The listing builds one solid part. Answer for the finished solid, in the listing's coordinates (mm). A direction names the side the tool comes from. Give positions to 0.01 mm unless a question says otherwise; leave off trailing zeros. Write each loop counter-clockwise with the first axis right and the second up, starting at its lowest first coordinate (ties: lowest second). Pieces come first, ordered by that corner, then holes. Notation, with made-up numbers: M 18.25,20 L 46.25,20 A32 ccw 46.25,57 Z; hole C -15,79 d4. An arc over 180 degrees is marked long. Answer as a JSON object with one key per item and string values.
Autodesk Inventor part; units mm, degrees
ref_plane "MSC_PF1" through (0, 0, 0) normal (1, 0, 0) x (0, 1, 0)
ref_plane "MSC_PT1" through (0, 0, 0) normal (0, 0, -1) x (-1, 0, 0)
ref_plane "YZ Plane" through (0, 0, 0) normal (1, 0, 0) x (0, 1, 0)
sketch "Esquisse1" plane through (0, 0, 0) normal (0, 1, 0) x (-1, 0, 0)
  point P0 (0, 0)
sketch "Esquisse2" plane through (0, 0, 0) normal (0, 0, 1) x (1, 0, 0)
  point P0 (0, 0)
sketch "Esquisse3" plane through (0, 0, 0) normal (0, 0, 1) x (1, 0, 0)
  point P0 (0, 0)
sketch "Esquisse4" plane through (0, 0, 0) normal (0, 1, 0) x (-1, 0, 0)
  line L0 (-3.65, 0) -> (0, 0)
  line L1 (-3.65, -0.45) -> (-3.65, 0)
  line L2 (-1.75, -2.35) -> (-3.65, -0.45)
  line L3 (-1.75, -2.65) -> (-1.75, -2.35)
  line L4 (-1.45, -2.95) -> (-1.75, -2.65)
  line L5 (-1.75, -3.25) -> (-1.45, -2.95)
  line L6 (-1.75, -10) -> (-1.75, -3.25)
  line L7 (0, 0) -> (0, -10)
  line L8 (0, 3.3392) -> (0, -10.7) construction
  line L9 (0, 3.3392) -> (0, -10.7)
  line L10 (0, -13.5078) -> (0, 6.1471)
  line L11 (-1.75, -10) -> (0, -10)
  line L12 (0.73, 0) -> (-4.38, 0)
  dimension "d3" = 3.65
  dimension "d5" = 0.3
  dimension "d7" = 0.3
  dimension "d9" = 0.3
  dimension "d11" = 2.35
  dimension "d13" = 135
  dimension "d17" = 1.45
  dimension "d19" = 0
  dimension "d51" = 1.75
  dimension "d52" = 10
revolve "Révolution1" add sketch "Esquisse4" angle 360 about axis through (0, 0, 3.3392) along (0, 0, -1)
sketch "Esquisse5" plane through (0, 0, 0) normal (0, 1, 0) x (-1, 0, 0)
  line L0 (-2.2, 0) -> (0, 0)
  line L1 (-0.3667, -2.1364) -> (-2.2, 0)
  line L2 (0, -2.1364) -> (-0.3667, -2.1364)
  line L3 (0, 0) -> (0, -2.1364)
  line L4 (-1.75, -2.35) -> (1.75, -2.35) construction
  line L5 (-3.65, 0) -> (3.65, 0)
  line L6 (0, -2.82) -> (0, 0.47)
  dimension "d22" = 2.2
  dimension "d24" = 0.3667
  dimension "d26" = 2.1364
extrude "Extrusion1" cut sketch "Esquisse5" along normal mid plane 0.7333
pattern_circular "RéseauPolaire1" count 4 over 360 about axis through (0, 0, 0) along (0, 0, 1) of "Extrusion1"
sketch "Esquisse7" plane through (0, 0, 0) normal (0, 1, 0) x (-1, 0, 0)
  line L0 (0, -1.175) -> (-2.75, 0)
  line L1 (0, 0) -> (0, -1.175)
  line L2 (-2.75, 0) -> (0, 0)
  line L3 (-1.75, -2.35) -> (1.75, -2.35) construction
  line L4 (0, -2.82) -> (0, 0.47)
  line L5 (-3.65, 0) -> (3.65, 0)
  dimension "d33" = 2.75
  dimension "d35" = 1.175
extrude "Extrusion2" cut sketch "Esquisse7" along normal mid plane 0.7333
pattern_circular "RéseauPolaire2" count 4 over 360 about axis through (0, 0, 0) along (0, 0, 1) of "Extrusion2"
fillet "Congé1" radius 0.6 1 edges at (-1.75, 0, -2.35)
thread "Filetage1"
ref_plane "MSC_PF1" through (0, 0, 0) normal (1, 0, 0) x (0, 1, 0)
ref_plane "MSC_PT1" through (0, 0, 0) normal (0, 0, -1) x (-1, 0, 0)
equation "\"d3\" = 0.5 * Dh"
equation "\"d5\" = msp_x"
equation "\"d7\" = ParA"
equation "\"d9\" = msp_x"
equation "\"d11\" = ParK"
equation "\"d17\" = 0.5 * msp_mdtds"
equation "\"d51\" = 0.5 * NND"
equation "\"d52\" = NLG"
equation "\"d22\" = 0.5 * M"
equation "\"d24\" = 0.0833333 * M"
equation "\"d26\" = 0.909091 * ParK"
equation "\"d27\" = 0.166667 * M"
equation "\"d33\" = 0.625 * M"
equation "\"d35\" = 0.5 * ParK"
equation "\"d36\" = 0.166667 * M"
equation "\"d41\" = 2 * msp_x"
equation "\"PTC\" = 0.6"
equation "\"NLG\" = 10"
equation "\"ParK\" = 2.35"
equation "\"NND\" = 3.5"
equation "\"M\" = 4.4"
equation "\"msp_mdtds\" = NND - PTC"
equation "\"Dh\" = 7.3"
equation "\"msp_x\" = 0.5 * PTC"
equation "\"ParA\" = 0.5 * PTC"
equation "\"r\" = 0.9"
equation "\"THREADDIA\" = NND"
equation "\"TEMPLATE\" = 1.2345"
properties part number "NF EN ISO 7046-2 H - M3.5x10 - 8.8 - H1" material "Acier inoxydable 440C"
1. A cutting plane is placed at A-A, the plane z = -6.75. Give the vertices of the cut face in (x, y).
Verdict:
{"outline": "C 0,0 d3.5"}
2. For faces 4 (the flat face through (0, 0, -10)), 5 (the flat face through (0.01, 1.11, -1.27)), 6 (the cylindrical face through (1.617, -0.67, -6.578)), determine the directions among +Z, -Z, +X, -X, +Y, -Y from which every point of the face is accessible in a straight line to the end or side of a thin tool.
Verdict:
{"face 4": "-Z, +X, -X, +Y, -Y", "face 5": "+Z", "face 6": "-Z"}
3. The mould has two halves that part along X. Classify faces 1 (the flat face through (-0.367, -1, -1)), 2 (the conical face through (-0.441, -1.985, -2.066)), 3 (the flat face through (1, 1, 0)): released by +X, released by -X, zero draft, split by the parting line, or undercut.
Verdict:
{"face 1": "undercut", "face 2": "split by the parting line", "face 3": "zero draft"}
4. Flat-ended cylindrical pins translate along their axes: pin 1 (2.5 mm diameter, centred on x = 2, z = -1.5, fed in from +Y); pin 2 (1.1 mm diameter, centred on y = 2, z = -1, fed in from -X); pin 3 (0.6 mm diameter, centred on x = 0, y = 0, fed in from +Z). Find the tip coordinate at first contact, or state that the pin passes through.
Verdict:
{"pin 1": "stops at y = 3.4", "pin 2": "stops at x = -3.13", "pin 3": "stops at z = -2.14"}
5. Consider line 1 along Z through (x, y) = (1.25, 1); line 2 along Y through (x, z) = (0.5, -5.25); line 3 along X through (y, z) = (0.75, -7). Determine where each line is inside the solid, lowest interval first.
Verdict:
{"line 1": "z = -10 to -3.1, -2.8 to 0", "line 2": "y = -1.68 to 1.68", "line 3": "x = -1.58 to 1.58"}
